```python
from build123d import *

# Parameters (mm, degrees)
SKETCH1_R           = 1.75
BOSS_EXTRUDE1_DEPTH = 8.5
BOSS_EXTRUDE2_START = -8.5
BOSS_EXTRUDE2_DEPTH = 8.5
FILLET1_R           = 7.5


with BuildPart() as part:
    # Sketch1 → Boss-Extrude1 (new body)
    with BuildSketch(Plane(origin=(0, 0, 0), x_dir=(0, 0, -1), z_dir=(1, 0, 0))):
        with BuildLine():
            Line((27, 10), (5, 10))
            ThreePointArc((5, 10), (0, 5), (5, 0))
            Line((5, 0), (27, 0))
            ThreePointArc((27, 0), (32, 5), (27, 10))
        make_face()
        with Locations((5, 5)):
            Circle(SKETCH1_R, mode=Mode.SUBTRACT)
        with Locations((27, 5)):
            Circle(SKETCH1_R, mode=Mode.SUBTRACT)
    extrude(amount=BOSS_EXTRUDE1_DEPTH)

    # Sketch2 → Boss-Extrude2 (add)
    with BuildSketch(Plane(origin=(8.5, 0, 0), x_dir=(0, 0, -1), z_dir=(1, 0, 0)).offset(BOSS_EXTRUDE2_START)):
        with BuildLine():
            Line((48.857901547, 17.499285579), (27, 10))
            ThreePointArc((27, 10), (31.900318254, 5.993418847), (28.947227404, 0.394752402))
            Line((28.947227404, 0.394752402), (51.973465393, 10.130889422))
            Line((51.973465393, 10.130889422), (48.857901547, 17.499285579))
        make_face()
    extrude(amount=BOSS_EXTRUDE2_DEPTH)

    # Fillet1
    fillet1_edges = [part.edges().sort_by_distance(p)[0] for p in [
        (4.25, 10, -27),
        (4.25, 17.499285579, -48.857901547),
    ]]
    fillet(fillet1_edges, radius=FILLET1_R)


solid = part.part
```
Read the model definition and answer for the solid it produces. Units are mm, in the model's axes. A direction names the side the tool comes from. Coordinates: 2 decimals unless noted, no trailing zeros. Loops run counter-clockwise (first coordinate to the right, second up) from the corner with the lowest first, then second, coordinate; pieces in that order, holes last. Notation, with made-up numbers: (-28.75, 67.25) - (17.25, 67.25) arc R9 ccw to (17.25, 76.25) - close; hole circle Ø7 at (81, 18.5). An arc over 180 degrees is marked (long way). Answer in a Markdown table with one row per item.
1. Find section C-C, the plane z = -22. Write down the section's boundary in (x, y).
Conclusion:
| item | result |
|---|---|
| outline | (0, 0) - (8.5, 0) - (8.5, 10) - (0, 10) - close |
2. Straight lines are drawn through the part: line 1 (Y direction, x = 5, z = -5); line 2 (Z direction, x = 7.25, y = 6.25); line 3 (Y direction, x = 6.75, z = -27). For each, find the intervals that lie inside material, in ascending order.
Conclusion:
| item | result |
|---|---|
| line 1 | y = 0 to 3.25, 6.75 to 10 |
| line 2 | z = -42.8 to -28.22, -25.78 to -6.22, -3.78 to -0.16 |
| line 3 | y = 0 to 3.25, 6.75 to 10.11 |
3. Which of the six approach directions +Z, -Z, +X, -X, +Y, -Y give full straight-line access (tool end or side, diameter ignored) to faces 1 (the face through (4, 5, 0)), 2 (the face through (4, 10, -16))?
Conclusion:
| item | result |
|---|---|
| face 1 | +Z, +X, -X |
| face 2 | +Z, +X, -X, +Y |
4. Find section A-A, the plane x = 3.25. Write down the section's boundary in (y, z), then the cut area to 3 significant figures.
Conclusion:
| item | result |
|---|---|
| outline | (0, -27) arc R5 ccw to (0.39, -28.95) - (10.13, -51.97) - (11.06, -51.58) arc R7.5 ccw to (15.23, -42.24) - (10.41, -28.18) arc R7.5 cw to (10, -25.75) - (10, -5) arc R5 ccw to (0, -5) - close; hole circle Ø3.5 at (5, -27); hole circle Ø3.5 at (5, -5) |
| area | 452 mm² |
5. Given pin 1 (2 mm diameter, centred on x = 7, z = -18, fed in from +Y); pin 2 (5.5 mm diameter, centred on y = 5, z = -27, fed in from -X); pin 3 (2 mm diameter, centred on x = 2, y = 3, fed in from -Z); pin 4 (1.5 mm diameter, centred on x = 3.5, z = -40, fed in from -Y), each flat-ended and moving along its own axis, determine where each tip first touches the part or whether it passes through.
Conclusion:
| item | result |
|---|---|
| pin 1 | stops at y = 10 |
| pin 2 | stops at x = 0 |
| pin 3 | stops at z = -37.47 |
| pin 4 | stops at y = 4.75 |
6. Find section B-B, the plane y = 4.25. Write down the section's boundary in (x, z) (3 decimals), then the cut area to 3 significant figures.
Conclusion:
| item | result |
|---|---|
| outline | (0, -38.065) - (8.5, -38.065) - (8.5, -28.581) - (0, -28.581) - close; (0, -25.419) - (8.5, -25.419) - (8.5, -6.581) - (0, -6.581) - close; (0, -3.419) - (8.5, -3.419) - (8.5, -0.057) - (0, -0.057) - close |
| area | 269 mm² |
7. Find section D-D, the plane y = 7.5. Write down the section's boundary in (x, z), then the cut area to 3 significant figures.
Conclusion:
| item | result |
|---|---|
| outline | (0, -45.75) - (8.5, -45.75) - (8.5, -0.67) - (0, -0.67) - close |
| area | 383 mm² |
8. Determine the mould class of faces 3 (the face through (0, 8, -26)), 4 (the face through (4.2, 0.1, -28)), 5 (the face through (4.19, 3.94, -3.61)) for opening direction Z: +Z half, -Z half, draft (parallel to the pull), parting line (faces both ways), or undercut.
Conclusion:
| item | result |
|---|---|
| face 3 | draft |
| face 4 | -Z half |
| face 5 | undercut |
